Verification items for the finished model (mm, model axes). A direction names the side the tool comes from. Coordinates: 2 decimals unless noted, no trailing zeros. Write each loop counter-clockwise with the first axis right and the second up, starting at its lowest first coordinate (ties: lowest second). Pieces come first, ordered by that corner, then holes. Notation, with made-up numbers: M 68,87.25 L 101,87.25 A17 cw 101,113.25 Z; hole C 24,3 d2. An arc over 180 degrees is marked long. Answer in a Markdown table with one row per item.
from build123d import *

# Parameters (mm, degrees)
F0_W     = 20
F0_H     = 50
F1_DEPTH = 5
F2_W     = 15
F2_H     = 4
F3_DEPTH = 5


with BuildPart() as f1:
    # F0 (on Top) → F1 (new body)
    with BuildSketch(Plane.XY):
        Rectangle(F0_W, F0_H)
        with BuildLine():
            ThreePointArc((-10, 25), (-21.477274, 0), (-10, -25))
            Line((-10, -25), (-10, 25))
        make_face()
    extrude(amount=F1_DEPTH)

    # F2 (on face) → F3 (join)
    with BuildSketch(Plane.XY.offset(5)):
        with Locations((2.5, 15)):
            Rectangle(F2_W, F2_H)
        with Locations((2.5, -15)):
            Rectangle(F2_W, F2_H)
    extrude(amount=F3_DEPTH)


solid = f1.part
1) Release check for a two-part mould opening along Y. For faces 4 (the face through (-5, -15, 7)), 5 (the face through (0, -25, 2)), 6 (the face through (-6, 0, 5)) record: +Y half, -Y half, draft (parallel to the pull), parting line (faces both ways), or undercut.
Response values:
| item | result |
|---|---|
| face 4 | draft |
| face 5 | -Y half |
| face 6 | undercut |
2) Sectioned sample at C-C (y = -21). Record the cut outline in (x, z), then the cut area to 3 significant figures.
Response values:
| item | result |
|---|---|
| outline | M -13.92,0 L 10,0 L 10,5 L -13.92,5 Z |
| area | 120 mm² |
3) Sectioned sample at B-B (x = 8.5). Record the cut outline in (y, z).
Response values:
| item | result |
|---|---|
| outline | M -25,0 L 25,0 L 25,5 L 17,5 L 17,10 L 13,10 L 13,5 L -13,5 L -13,10 L -17,10 L -17,5 L -25,5 Z |
4) Thickness scan on L1, parallel to Y at x = -3, z = 6.25; L2, parallel to Z at x = -9, y = 14; L3, parallel to X at y = 16.5, z = 6.5. Record the ranges inside material, lowest first. Write a range as [from, to].
Response values:
| item | result |
|---|---|
| L1 | y = [-17, -13], [13, 17] |
| L2 | z = [0, 5] |
| L3 | x = [-5, 10] |
5) Sectioned sample at D-D (x = -7). Record the cut outline in (y, z), then the cut area to 3 significant figures.
Response values:
| item | result |
|---|---|
| outline | M -25,0 L 25,0 L 25,5 L -25,5 Z |
| area | 250 mm² |
6) Tool access check on faces 1 (the face through (2, 17, 7)), 2 (the face through (-5, 15, 7)), 3 (the face through (2, 13, 7)). Record the directions out of +Z, -Z, +X, -X, +Y, -Y that give a thin tool (end or side, any length) a straight path to the whole face; none if there is none.
Response values:
| item | result |
|---|---|
| face 1 | +Z, +X, -X, +Y |
| face 2 | +Z, -X, +Y, -Y |
| face 3 | +Z, +X, -X |
7) Depth check by flat-ended pin: pin 1 (1.5 mm diameter, centred on x = -1, z = 7.5, fed in from -Y); pin 2 (1.2 mm diameter, centred on y = -15.5, z = 7.5, fed in from -X); pin 3 (4 mm diameter, centred on x = 4, z = 8, fed in from +Y). Enter the tip coordinate at first touch or a pass-through.
Response values:
| item | result |
|---|---|
| pin 1 | stops at y = -17 |
| pin 2 | stops at x = -5 |
| pin 3 | stops at y = 17 |
8) Sectioned sample at A-A (z = 5.5). Record the cut outline in (x, y).
Response values:
| item | result |
|---|---|
| outline | M -5,-17 L 10,-17 L 10,-13 L -5,-13 Z; M -5,13 L 10,13 L 10,17 L -5,17 Z |
